The listing builds one solid part. Answer for the finished solid, in the listing's coordinates (mm). Face numbers are marked on the shaded views. Give positions to 0.01 mm unless a question says otherwise; leave off trailing zeros. Order: outer loops, then holes, each group sorted by start corner. A loop starts at its lowest first (then second) coordinate and runs counter-clockwise, first axis right, second up. Notation, with made-up numbers: (-6, -4) - (2, -4) arc R10 ccw to (2, 5) - close; hole circle Ø1 at (35, 38). An arc over 180 degrees is marked (long way). Answer in a Markdown table with one row per item.
from build123d import *

# Parameters (mm, degrees)
F0_W     = 85
F0_H     = 23
F1_DEPTH = 3
F2_W     = 3
F2_H     = 23
F3_DEPTH = 24
F4_W     = 3
F4_H     = 23
F5_DEPTH = 25


with BuildPart() as f1:
    # F0 (on Top) → F1 (new body)
    with BuildSketch(Plane.XY):
        with Locations((42.5, 11.5)):
            Rectangle(F0_W, F0_H)
        with BuildLine():
            Line((85, 0), (0, 0))
            Line((0, 0), (0, -10))
            Line((0, -10), (0, -65))
            ThreePointArc((0, -65), (1.464466, -68.535534), (5, -70))
            Line((5, -70), (7.5, -70))
            ThreePointArc((7.5, -70), (11.035534, -68.535534), (12.5, -65))
            Line((12.5, -65), (12.5, -15))
            ThreePointArc((12.5, -15), (13.964466, -11.464466), (17.5, -10))
            Line((17.5, -10), (67.5, -10))
            ThreePointArc((67.5, -10), (71.035534, -11.464466), (72.5, -15))
            Line((72.5, -15), (72.5, -65))
            ThreePointArc((72.5, -65), (73.964466, -68.535534), (77.5, -70))
            Line((77.5, -70), (80, -70))
            ThreePointArc((80, -70), (83.535534, -68.535534), (85, -65))
            Line((85, -65), (85, -10))
            Line((85, -10), (85, 0))
        make_face()
    extrude(amount=F1_DEPTH)

    # F2 (on face) → F3 (join)
    with BuildSketch(Plane.XY.offset(3)):
        with Locations((1.5, 11.5)):
            Rectangle(F2_W, F2_H)
        with Locations((83.5, 11.5)):
            Rectangle(F2_W, F2_H)
    extrude(amount=F3_DEPTH)

    # F4 (on face) → F5 (join)
    with BuildSketch(Plane.XY.offset(27)):
        with Locations((1.5, 11.5)):
            Rectangle(F4_W, F4_H)
    extrude(amount=F5_DEPTH)


solid = f1.part
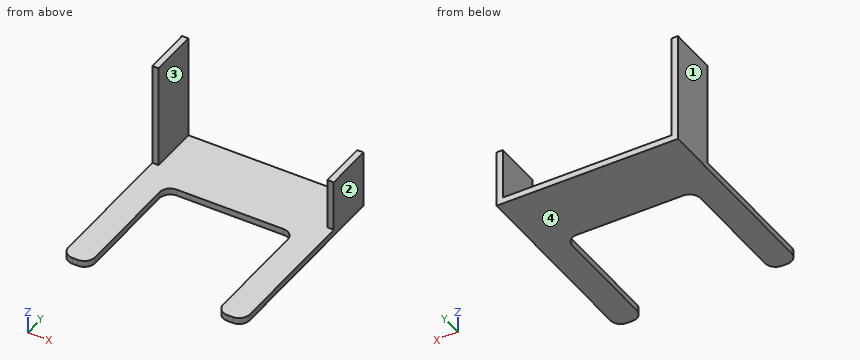
Item 1: Determine the mould class of the marked faces 1, 2, 3 and 4 for opening direction X: pulls with the +X half, pulls with the -X half, needs draft (parallel to the pull), parting line crosses it, or undercut.
Answer block:
| item | result |
|---|---|
| face 1 | pulls with the -X half |
| face 2 | pulls with the +X half |
| face 3 | undercut |
| face 4 | needs draft |
Item 2: Each of these flat-tipped pins is pushed along its axis until it touches: P1, Ø1.5, axis at x = 83, z = 10.5, coming from the -Y side; P2, Ø0.9, axis at x = 83, y = 11.5, coming from the +Z side; P3, Ø11.5, axis at y = 15, z = 20.5, coming from the -X side; P4, Ø6, axis at y = 7, z = 37, coming from the +X side. Where does it stop, or does it pass through?
Answer block:
| item | result |
|---|---|
| P1 | y = 0 |
| P2 | z = 27 |
| P3 | x = 0 |
| P4 | x = 3 |
Item 3: Consider line 1 (X direction, y = 12, z = 23.5); line 2 (Z direction, x = 5, y = -37). Determine where each line is inside the solid, lowest interval first.
Answer block:
| item | result |
|---|---|
| line 1 | 0 to 3, 82 to 85 |
| line 2 | 0 to 3 |
Item 4: Find section A-A on y = -29. Write down the section's boundary in (x, z), then the cut area to 3 significant figures.
Answer block:
| item | result |
|---|---|
| outline | (0, 0) - (12.5, 0) - (12.5, 3) - (0, 3) - close; (72.5, 0) - (85, 0) - (85, 3) - (72.5, 3) - close |
| area | 75.0 mm² |
Item 5: Find section D-D on z = 45.5. Write down the section's boundary in (x, y).
Answer block:
| item | result |
|---|---|
| outline | (0, 0) - (3, 0) - (3, 23) - (0, 23) - close |
Item 6: Find section B-B on z = 16. Write down the section's boundary in (x, y), then the cut area to 3 significant figures.
Answer block:
| item | result |
|---|---|
| outline | (0, 0) - (3, 0) - (3, 23) - (0, 23) - close; (82, 0) - (85, 0) - (85, 23) - (82, 23) - close |
| area | 138 mm² |
Item 7: Find section C-C on y = 15.5. Write down the section's boundary in (x, z), then the cut area to 3 significant figures.
Answer block:
| item | result |
|---|---|
| outline | (0, 0) - (85, 0) - (85, 27) - (82, 27) - (82, 3) - (3, 3) - (3, 52) - (0, 52) - close |
| area | 474 mm² |
